The model under review builds one solid part; all positions refer to its coordinate system, in mm. A direction names the side the tool comes from. Coordinates: 2 decimals unless noted, no trailing zeros. Loops run counter-clockwise (first coordinate to the right, second up) from the corner with the lowest first, then second, coordinate; pieces in that order, holes last. Notation, with made-up numbers: (30, 75) - (61, 75) arc R16 ccw to (61, 93) - close; hole circle Ø4 at (24.5, -1.75). An arc over 180 degrees is marked (long way). Answer in a Markdown table with one row per item. Add a question column.
(1) We need section B-B on y = 40. Write out the cut boundary in (x, z) (3 decimals).
(2) For P1, Ø15.5, axis at x = 53.5, z = 45, coming from the -Y side; P2, Ø5, axis at y = 12.5, z = 19, coming from the -X side (3 decimals); P3, Ø5, axis at x = 55, y = 7.5, coming from the +Z side; P4, Ø14, axis at y = -21, z = 16, coming from the -X side (3 decimals), all flat-tipped, find the tip position at first contact; note any pin that passes through.
(3) We need section A-A on x = 73.5. Write out the cut boundary in (y, z) (1 decimal).
(4) For line 1 along Y through (x, z) = (-31.5, 26); line 2 along X through (y, z) = (-9.5, -3) (3 decimals); line 3 along Z through (x, y) = (104.5, 3) (3 decimals), list the stretches that pass through material, from the lowest coordinate up.
(5) Mouldability with a two-part tool opening along X and no side actions: class faces 5 (the flat face through (86, 0, 66.675)), 6 (the flat face through (60.325, 0, 41)), 7 (the flat face through (22.225, -17, 18)) as +X half, -X half, draft (parallel to the pull), parting line (faces both ways), or undercut.
(6) Machinability: for faces 1 (the flat face through (47, -25.4, 42)), 2 (the flat face through (-4, -7.938, 30)), 3 (the cylindrical face through (45.8, -0.4, 38.1)), 4 (the flat face through (41.275, -1, 4)), which of the approach directions +Z, -Z, +X, -X, +Y, -Y give a long, thin tool a straight path to every point of the face, cutting with its end or side? Answer none if there is none.
(7) We need section C-C on z = 3. Write out the cut boundary in (x, y) (3 decimals), plus the area to 3 significant figures.
from build123d import *

# Parameters (mm, degrees)
F1_DEPTH = 63.5
F2_DEPTH = 25.4
F3_DEPTH = 7.9375


with BuildPart() as f1:
    # F0 (on Front) → F1 (new body, symmetric)
    with BuildSketch(Plane.XZ):
        Polygon((41.275, -9.525), (41.275, 9.525), (22.225, 9.525), (-41.275, 9.525), (-41.275, -9.525), align=None)
    extrude(amount=F1_DEPTH, both=True)

    # F0 (on Front) → F2 (join, symmetric)
    with BuildSketch(Plane.XZ):
        with BuildLine():
            Line((22.225, 9.525), (41.275, 9.525))
            Line((41.275, 9.525), (41.275, 27.0002))
            ThreePointArc((41.275, 27.0002), (45.9246798487, 38.2255201513), (57.15, 42.8752))
            Line((57.15, 42.8752), (60.325, 42.8752))
            Line((60.325, 42.8752), (60.325, 61.9252))
            Line((60.325, 61.9252), (57.15, 61.9252))
            add(Edge.make_bspline(
                [(55.5210256517, 61.8871899471), (56.0671839511, 61.9033086419), (56.6102374814, 61.9159842015), (57.15, 61.9252)],
                knots=[110.0017210547, 110.0017210547, 110.0017210547, 110.0017210547, 111.5045361635, 111.5045361635, 111.5045361635, 111.5045361635], degree=3))
            ThreePointArc((55.5210256517, 61.8871899471), (31.8849297041, 51.1130979582), (22.225, 27.0002))
            Line((22.225, 27.0002), (22.225, 9.525))
        make_face()
        Polygon((60.325, 61.9252), (60.325, 42.8752), (85.7483517106, 42.8752), (85.8415101305, 61.9252), align=None)
    extrude(amount=F2_DEPTH, both=True)

    # F0 (on Front) → F3 (join, symmetric)
    with BuildSketch(Plane.XZ):
        Polygon((41.275, -9.525), (41.275, 9.525), (22.225, 9.525), (-41.275, 9.525), (-41.275, -9.525), align=None)
        with BuildLine():
            Line((22.225, 9.525), (41.275, 9.525))
            Line((41.275, 9.525), (41.275, 27.0002))
            ThreePointArc((41.275, 27.0002), (45.9246798487, 38.2255201513), (57.15, 42.8752))
            Line((57.15, 42.8752), (60.325, 42.8752))
            Line((60.325, 42.8752), (60.325, 61.9252))
            Line((60.325, 61.9252), (57.15, 61.9252))
            add(Edge.make_bspline(
                [(55.5210256517, 61.8871899471), (56.0671839511, 61.9033086419), (56.6102374814, 61.9159842015), (57.15, 61.9252)],
                knots=[110.0017210547, 110.0017210547, 110.0017210547, 110.0017210547, 111.5045361635, 111.5045361635, 111.5045361635, 111.5045361635], degree=3))
            ThreePointArc((55.5210256517, 61.8871899471), (31.8849297041, 51.1130979582), (22.225, 27.0002))
            Line((22.225, 27.0002), (22.225, 9.525))
        make_face()
        with BuildLine():
            Line((-41.275, 9.525), (22.225, 9.525))
            Line((22.225, 9.525), (22.225, 27.0002))
            ThreePointArc((22.225, 27.0002), (31.8849297041, 51.1130979582), (55.5210256517, 61.8871899471))
            add(Edge.make_bspline(
                [(-41.275, 9.525), (-41.0681757543, 41.079819722), (15.5438171721, 60.7073480966), (55.5210256517, 61.8871899471)],
                knots=[0, 0, 0, 0, 110.0017210547, 110.0017210547, 110.0017210547, 110.0017210547], degree=3))
        make_face()
        Polygon((85.7483517106, 42.8752), (60.325, 42.8752), (60.325, 38.1), (85.725, 38.1), align=None)
        Polygon((60.325, 61.9252), (60.325, 42.8752), (85.7483517106, 42.8752), (85.8415101305, 61.9252), align=None)
        Polygon((60.325, 66.675), (60.325, 61.9252), (85.8415101305, 61.9252), (85.8647376299, 66.675), align=None)
        Polygon((85.8415101305, 61.9252), (85.7483517106, 42.8752), (85.725, 38.1), (111.125, 38.1), (111.125, 66.675), (85.8647376299, 66.675), align=None)
    extrude(amount=F3_DEPTH, both=True)


solid = f1.part
Outcome:
| question | item | result |
|---|---|---|
| 1 | outline | (-41.275, -9.525) - (41.275, -9.525) - (41.275, 9.525) - (-41.275, 9.525) - close |
| 2 | P1 | y = -25.4 |
| 2 | P2 | x = 22.225 |
| 2 | P3 | z = 61.93 |
| 2 | P4 | x = -41.275 |
| 3 | outline | (-25.4, 42.9) - (-7.9, 42.9) - (-7.9, 38.1) - (7.9, 38.1) - (7.9, 42.9) - (25.4, 42.9) - (25.4, 61.9) - (7.9, 61.9) - (7.9, 66.7) - (-7.9, 66.7) - (-7.9, 61.9) - (-25.4, 61.9) - close |
| 4 | line 1 | -7.94 to 7.94 |
| 4 | line 2 | -41.275 to 41.275 |
| 4 | line 3 | 38.1 to 66.675 |
| 5 | face 5 | draft |
| 5 | face 6 | undercut |
| 5 | face 7 | -X half |
| 6 | face 1 | +Z, +X, -X, -Y |
| 6 | face 2 | +Z, -X, -Y |
| 6 | face 3 | -Z, +Y, -Y |
| 6 | face 4 | -Z, +X, +Y, -Y |
| 7 | outline | (-41.275, -63.5) - (41.275, -63.5) - (41.275, 63.5) - (-41.275, 63.5) - close |
| 7 | area | 10,500 mm² |
